For this review, take the finished solid that the model builds, in its own axes (mm). A direction names the side the tool comes from. Give positions to 0.01 mm unless a question says otherwise; leave off trailing zeros. Loops run counter-clockwise (first coordinate to the right, second up) from the corner with the lowest first, then second, coordinate; pieces in that order, holes last. Notation, with made-up numbers: (51.25, 78.25) -> (85.25, 78.25) arc R8 ccw to (85.25, 85.25) -> close; hole circle Ø3 at (38, 20). An arc over 180 degrees is marked (long way). One line per question, with ' | ' between items. Start each with the question number.
(1) Consider section B-B (y = -0.9). Write out the cut boundary in (x, z).
(2) Consider section D-D (z = 9). Write out the cut boundary in (x, y), and give its area (3 significant figures).
(3) Tool access review of faces 1 (the cylindrical face through (24.87, -2.52, -0.33)), 2 (the flat face through (19, 2.54, 6)): name each direction out of +Z, -Z, +X, -X, +Y, -Y from which nothing blocks a thin tool from reaching the whole face with its end or side.
(4) Wall thickness on probe 1 along Z at (x, y) = (-6.5, 0.8); probe 2 along X at (y, z) = (-0.8, 9.25); probe 3 along X at (y, z) = (-0.8, 3.75): over which ranges is each line inside the solid? List them lowest first.
(5) Insertion check: P1, Ø1.5, axis at y = 0.5, z = 7.5, coming from the +X side; P2, Ø1, axis at y = 2, z = 11, coming from the -X side; P3, Ø1.5, axis at y = -0.5, z = 9.5, coming from the -X side. Each pin has a flat end and moves straight along its axis. Give the tip position at first contact, or say it passes through.
(6) Consider section A-A (z = 4.75). Write out the cut boundary in (x, y).
(7) Consider section C-C (x = 6). Write out the cut boundary in (y, z).
(8) Draft analysis for pull direction X (two halves, no side actions). For faces 3 (the flat face through (-6, 2.54, 6)), 4 (the flat face through (-5.335, -0.036, 7.672)), 5 (the flat face through (63.5, 0, 0)), state which applies: +X half, -X half, draft (parallel to the pull), parting line (faces both ways), or undercut.
from build123d import *

# Parameters (mm, degrees)
F2_DEPTH = 2.54
F1_W     = 2.54
F1_H     = 12.7
F0_W     = 63.5
F0_H     = 2.54
F0_W_2   = 12.7


with BuildPart() as f2:
    # F1 (on Front) → F2 (new body, symmetric)
    with BuildSketch(Plane.XZ):
        Polygon((-3.4942510538, 0), (0, 0), (-8.8303433731, 12.7), (-11.3703433731, 12.7), align=None)
    extrude(amount=F2_DEPTH, both=True)



with BuildPart() as f2b:
    # F1 (on Front) → F2, piece 2 (new body, symmetric)
    with BuildSketch(Plane.XZ):
        with Locations((18.6417625439, 6.35)):
            Rectangle(F1_W, F1_H)
    extrude(amount=F2_DEPTH, both=True)


with BuildPart() as f2_1:
    add(f2.part)

    add(f2b.part)  # F3 merges F2b
    # F0 (on Front) → F3 (revolve)
    with BuildSketch(Plane.XZ):
        with Locations((31.75, 1.27)):
            Rectangle(F0_W, F0_H)
        with Locations((-6.35, 1.27)):
            Rectangle(F0_W_2, F0_H)
    revolve(axis=Axis((31.75, 0, 0), (1, 0, 0)))


solid = f2_1.part
A:
1) outline: (-12.7, -2.38) -> (63.5, -2.38) -> (63.5, 2.38) -> (19.91, 2.38) -> (19.91, 12.7) -> (17.37, 12.7) -> (17.37, 2.38) -> (-1.65, 2.38) -> (-8.83, 12.7) -> (-11.37, 12.7) -> (-4.97, 2.38) -> (-12.7, 2.38) -> close
2) outline: (-9.08, -2.54) -> (-6.26, -2.54) -> (-6.26, 2.54) -> (-9.08, 2.54) -> close; (17.37, -2.54) -> (19.91, -2.54) -> (19.91, 2.54) -> (17.37, 2.54) -> close | area: 27.2 mm^2
3) face 1: none | face 2: +Z, -Z, +X, -X, +Y
4) probe 1: z = -2.41 to 2.41, 4.85 to 9.35 | probe 2: x = -9.23 to -6.43, 17.37 to 19.91 | probe 3: x = -5.82 to -2.61, 17.37 to 19.91
5) P1: stops at x = 19.91 | P2: stops at x = -10.63 | P3: stops at x = -9.85
6) outline: (-6.44, -2.54) -> (-3.3, -2.54) -> (-3.3, 2.54) -> (-6.44, 2.54) -> close; (17.37, -2.54) -> (19.91, -2.54) -> (19.91, 2.54) -> (17.37, 2.54) -> close
7) outline: circle Ø5.08 at (0, 0)
8) face 3: draft | face 4: undercut | face 5: +X half
